Geometry check sheet. Reference: the model listing, model coordinates, mm. A direction names the side the tool comes from. Give positions to 0.01 mm unless a question says otherwise; leave off trailing zeros. Write each loop counter-clockwise with the first axis right and the second up, starting at its lowest first coordinate (ties: lowest second). Pieces come first, ordered by that corner, then holes. Notation, with made-up numbers: (-22, 20.5) - (16, 20.5) arc R28 cw to (16, 58.5) - close; hole circle Ø4 at (17, 64). An arc over 180 degrees is marked (long way). One line per question, with ' | ' between items. Start each with the question number.
Q1. Section check A-A on x = 0. Record the boundary of the cut face in (y, z), and give its area (3 significant figures).
Q2. Set-up check for faces 5 (the face through (0.1, 0.1, 25.5)), 6 (the face through (0, 97, 6.35)), 7 (the face through (0, 66, 19.05)): record each of +Z, -Z, +X, -X, +Y, -Y from which the full face is reachable in a straight line by a thin tool's end or side.
Q3. Section check C-C on z = 8. Record the boundary of the cut face in (x, y) (3 decimals).
Q4. Section check B-B on y = 82.5. Record the boundary of the cut face in (x, z), and give its area (3 significant figures).
Q5. Release check for a two-part mould opening along Y. For faces 1 (the face through (-16.77, -4.62, 29.64)), 2 (the face through (-3.65, -10.77, 23.73)), 3 (the face through (-19.05, 41, 3)), 4 (the face through (-0.27, 23.24, 29.1)) record: +Y half, -Y half, draft (parallel to the pull), parting line (faces both ways), or undercut.
Q6. Thickness scan on L1, parallel to Z at x = 2.5, y = 93; L2, parallel to Y at x = 4.5, z = 20.5; L3, parallel to Y at x = 0, z = 9. Record the ranges inside material, lowest first. Write a range as [from, to].
Q7. Section check D-D on x = -6. Record the boundary of the cut face in (y, z).
Q8. Gauge pin test, flat ends, axial feed: P1, Ø21, axis at x = -0.5, y = 99, coming from the +Z side; P2, Ø4, axis at x = 14.5, z = 24, coming from the +Y side; P3, Ø4, axis at x = -8, y = 1.5, coming from the +Z side. Record the tip position at first contact, or that the pin passes through.
```python
from build123d import *

# Parameters (mm, degrees)
SKETCH11_W          = 38.1
SKETCH11_H          = 38.1
SKETCH12_W          = 38.1
SKETCH12_H          = 38.1
BOSS_EXTRUDE5_DEPTH = 12.7
BOSS_EXTRUDE5_TAPER = 20
BOSS_EXTRUDE6_DEPTH = 38.1
SKETCH14_R          = 9.525
CUT_EXTRUDE2_DEPTH  = 12.7
SKETCH15_R          = 9.525
CUT_EXTRUDE3_DEPTH  = 12.7


with BuildPart() as part:
    # Sweep1: sweep along a path in Sketch10
    with BuildLine(Plane(origin=(0, 0, 0), x_dir=(0, 0, -1), z_dir=(1, 0, 0))) as sweep1_path:
        Line((0, 96.393), (0, 25.4))
        Line((0, 25.4), (-25.4, 0))
    # Sketch11 → Sweep1 (sweep)
    with BuildSketch(Plane(origin=(0, 96.393, 0), x_dir=(1, 0, 0), z_dir=(0, 1, 0))):
        Rectangle(SKETCH11_W, SKETCH11_H)
    sweep(path=sweep1_path.line, transition=Transition.RIGHT)

    # Sketch12 → Boss-Extrude5 (add)
    with BuildSketch(Plane(origin=(0, -12.7, 12.7), x_dir=(1, 0, 0), z_dir=(0, -0.7071067811865461, 0.7071067811865489))):
        with Locations((0, 17.960512242)):
            Rectangle(SKETCH12_W, SKETCH12_H)
    extrude(amount=BOSS_EXTRUDE5_DEPTH, taper=BOSS_EXTRUDE5_TAPER)

    # Sketch13 → Boss-Extrude6 (add)
    with BuildSketch(Plane(origin=(0, 0, -19.05), x_dir=(-1, 0, 0), z_dir=(0, 0, -1))):
        with BuildLine():
            Line((-19.05, 96.393), (19.05, 96.393))
            ThreePointArc((19.05, 96.393), (0, 115.443), (-19.05, 96.393))
        make_face()
    extrude(amount=-BOSS_EXTRUDE6_DEPTH)

    # Sketch14 → Cut-Extrude2 (cut)
    with BuildSketch(Plane.XY.offset(19.05)):
        with Locations((0, 96.393)):
            Circle(SKETCH14_R)
    extrude(amount=-CUT_EXTRUDE2_DEPTH, mode=Mode.SUBTRACT)

    # Sketch15 → Cut-Extrude3 (cut)
    with BuildSketch(Plane(origin=(0, -21.680256121, 21.680256121), x_dir=(1, 0, 0), z_dir=(0, -0.7071067811865461, 0.7071067811865489))):
        with Locations(Location((0, 17.960512242, 0), (0, 0, 270))):
            Circle(SKETCH15_R)
    extrude(amount=-CUT_EXTRUDE3_DEPTH, mode=Mode.SUBTRACT)


solid = part.part
```
Working result:
1) outline: (-19.18, 24.18) - (-13.47, 11.93) - (17.51, -19.05) - (115.44, -19.05) - (115.44, 19.05) - (105.92, 19.05) - (105.92, 6.35) - (86.87, 6.35) - (86.87, 19.05) - (33.29, 19.05) - (13.47, 38.87) - (1.22, 44.58) - (-2.25, 41.12) - (6.74, 32.14) - (-6.74, 18.66) - (-15.72, 27.65) - close | area: 4,740 mm2
2) face 5: none | face 6: +Z | face 7: +Z, +X, -X, +Y
3) outline: (-19.05, -9.541) - (19.05, -9.541) - (19.05, 96.393) arc R19.05 ccw to (-19.05, 96.393) - close; hole circle Ø19.05 at (0, 96.393)
4) outline: (-19.05, -19.05) - (19.05, -19.05) - (19.05, 19.05) - (-19.05, 19.05) - close | area: 1,450 mm2
5) face 1: -Y half | face 2: undercut | face 3: draft | face 4: +Y half
6) L1: z = [-19.05, 6.35] | L2: y = [-17.47, -6.97], [-4.9, 31.84] | L3: y = [-10.54, 86.87], [105.92, 115.44]
7) outline: (-19.18, 24.18) - (-13.47, 11.93) - (17.51, -19.05) - (114.47, -19.05) - (114.47, 19.05) - (103.79, 19.05) - (103.79, 6.35) - (89, 6.35) - (89, 19.05) - (33.29, 19.05) - (13.47, 38.87) - (1.22, 44.58) - (-3.75, 39.61) - (5.23, 30.63) - (-5.23, 20.17) - (-14.21, 29.15) - close
8) P1: stops at z = 19.05 | P2: stops at y = 30.34 | P3: stops at z = 44.58
